Here's how the part is built. I have some questions about the finished solid (model axes, mm). A direction names the side the tool comes from. Coordinates: 2 decimals unless noted, no trailing zeros. Write each loop counter-clockwise with the first axis right and the second up, starting at its lowest first coordinate (ties: lowest second). Pieces come first, ordered by that corner, then holes. Notation, with made-up numbers: M 82.25,4 L 123.25,4 A12 cw 123.25,21 Z; hole C 86,5.5 d11. An arc over 180 degrees is marked long. Write each question's results on one line, items separated by ' | '. Start each with the question number.
Autodesk Inventor part; units mm, degrees
ref_plane "YZ Plane" through (0, 0, 0) normal (1, 0, 0) x (0, 1, 0)
ref_plane "XZ Plane" through (0, 0, 0) normal (0, 1, 0) x (-1, 0, 0)
ref_plane "XY Plane" through (0, 0, 0) normal (0, 0, 1) x (1, 0, 0)
sketch "草圖1" plane through (0, 0, 0) normal (1, 0, 0) x (0, 1, 0)
  line L0 (-312, 12.65) -> (-317, 12.65)
  line L1 (-317, 12.65) -> (-317, -12.65)
  line L2 (-317, -12.65) -> (-312, -12.65)
  line L3 (-308, -12.65) -> (-308, 12.65) construction
  arc A0 (-310.3276, -7.5781) -> (-310.3276, 7.5781) centre (-321.5, 0) ccw
  line L4 (-310.5, -8.1394) -> (-310.5, -11.15)
  line L5 (-310.5, 8.1394) -> (-310.5, 11.15)
  arc A1 (-310.3276, -7.5781) -> (-310.5, -8.1394) centre (-309.5, -8.1394) ccw
  arc A2 (-310.5, 8.1394) -> (-310.3276, 7.5781) centre (-309.5, 8.1394) ccw
  arc A3 (-312, -12.65) -> (-310.5, -11.15) centre (-312, -11.15) ccw
  arc A4 (-310.5, 11.15) -> (-312, 12.65) centre (-312, 11.15) ccw
  line L6 (0, 0) -> (0, 24.9603) construction
  dimension "d0" = 317
  dimension "d1" = 9
  dimension "d2" = 12.65
  dimension "d3" = 25.3
  dimension "d4" = 27
  dimension "d5" = 0
  dimension "d6" = 2.5
  dimension "d7" = 2.5
  dimension "d8" = 2
  dimension "d9" = 2
  dimension "d10" = 3
  dimension "d11" = 3
revolve "迴轉1" add sketch "草圖1" angle 90 about axis through (0, 0, 0) along (0, 0, 1)
properties part number "異形橡膠圈-半圓"
1) For pin 1 Ø1 at (y, z) = (-86.5, 4) entering from -X; pin 2 Ø1.5 at (y, z) = (-233.5, 7) entering from -X; pin 3 Ø3 at (y, z) = (-111.5, -1.5) entering from -X, each with a flat end and sliding along its axis, tell me the tip position at first contact or that it passes through.
2) I want a section at A-A, the plane z = 0. Write out the boundary of the cut face in (x, y), then the cut area to 3 significant figures.
3) We'd pull the mould along X, two halves only. Please class faces 3 (the flat face through (314, 0, 0)), 4 (the cylindrical face through (226.604, -221.675, -0.177)), 5 (the cylindrical face through (217.129, -221.957, 9.666)): pulls with the +X half, pulls with the -X half, needs draft (parallel to the pull), parting line crosses it, or undercut.
4) For faces 1 (the flat face through (241, -205, -12.65)), 2 (the cylindrical face through (221.957, -217.129, -9.666)), which set-ups out of +Z, -Z, +X, -X, +Y, -Y let a thin tool reach every point of the face, with its end or its side?
5) Please list where these lines run through material, in increasing order: line 1 (Y direction, x = 183.5, z = 2); line 2 (X direction, y = -178, z = -4.5); line 3 (X direction, y = -20, z = -9.25). Write a range as [from, to].
Output:
1) pin 1: stops at x = 296.02 | pin 2: stops at x = 202.75 | pin 3: stops at x = 286.59
2) outline: M 0,-317 A317 ccw 317,0 L 308,0 A308 cw 0,-308 Z | area: 4,420 mm2
3) face 3: needs draft | face 4: pulls with the +X half | face 5: pulls with the -X half
4) face 1: -Z, +X, -X, +Y, -Y | face 2: -Z, -X, +Y
5) line 1: y = [-258.49, -247.56] | line 2: x = [252.3, 262.31] | line 3: x = [309.86, 316.37]
